The listing builds one solid part. Answer for the finished solid, in the listing's coordinates (mm). A direction names the side the tool comes from. Round coordinates to 2 decimals unless told otherwise and drop trailing zeros. Loops run counter-clockwise (first coordinate to the right, second up) from the corner with the lowest first, then second, coordinate; pieces in that order, holes last. Notation, with made-up numbers: (32, 59) - (42, 59) arc R13 cw to (42, 65) - close; hole circle Ø5 at (-15.75, -5). An arc over 180 degrees is marked (long way). Write item = value, one per line. Start each with the question number.
1) Section A-A, the plane x = -52 is taken. Determine the outline of the cut face in (y, z).
2) Section C-C, the plane z = 27 is taken. Determine the outline of the cut face in (x, y).
3) Given pin 1 Ø1.6 at (y, z) = (1, -34) entering from -X; pin 2 Ø1 at (x, z) = (-32, 20) entering from +Y; pin 3 Ø1.2 at (x, y) = (18.5, 1) entering from +Z; pin 4 Ø2 at (x, z) = (41, -18) entering from -Y, each flat-ended and moving along its own axis, determine where each tip first touches the part or whether it passes through.
4) A tool of negligible diameter and unlimited length cuts with its end or side. For faces 1 (the flat face through (42, 3.5, 36)), 2 (the flat face through (44.2, 1.7, -33)), 3 (the flat face through (52, 30, -35)), 4 (the flat face through (-50, 3.5, -36)), from which of +Z, -Z, +X, -X, +Y, -Y can it reach the whole face along a straight path? Write none if from no direction.
5) Section B-B, the plane y = 6 is taken. Determine the outline of the cut face in (x, z), and give its area (3 significant figures).
6) Section D-D, the plane y = 13.5 is taken. Give the number of separate pieces and of enclosed holes in the cut face, and give its area (3 significant figures).
7) Straight lines are drawn through the part: line 1 along Y through (x, z) = (-52, -36); line 2 along X through (y, z) = (38, 4.5); line 3 along X through (y, z) = (13, -36). For each, find the intervals that lie inside material, in ascending order.
8) For a pull along Y with two mould halves and no side action, classify faces 5 (the flat face through (46, 30, 0)), 6 (the flat face through (-42, 3.5, 36)), 7 (the cylindrical face through (-49.69, 12.54, -35.74)), 8 (the flat face through (-45, 57.5, -6)) as released by +Y, released by -Y, zero draft, split by the parting line, or undercut.
from build123d import *

# Parameters (mm, degrees)
SKETCH1_W                    = 89
SKETCH1_H                    = 70
BASE_FLANGE1_DEPTH           = 1.5
EDGE_FLANGE1_STRIP_W         = 10
EDGE_FLANGE1_STRIP_H         = 1.5
EDGE_FLANGE1_STRIP_CUT_DEPTH = 70
EDGE_FLANGE1_DEPTH           = 70
EDGE_FLANGE2_DEPTH           = 57.5
EDGE_FLANGE2_2_DEPTH         = 3.5
EDGE_FLANGE2_START           = 3.5
EDGE_FLANGE2_3_DEPTH         = 54
EDGE_FLANGE3_DEPTH           = 57.5
EDGE_FLANGE3_2_DEPTH         = 3.5
EDGE_FLANGE3_START           = 3.5
EDGE_FLANGE3_3_DEPTH         = 54
SKETCH16_R                   = 2.5
CUT_EXTRUDE1_DEPTH           = 10


# Read off the part's stored shape, not the designer's step: Edge-Flange2, Edge-Flange3
# Sheet-metal steps are written as plain solids
with BuildPart() as part:
    # Sketch1 → Base-Flange1 (new body)
    with BuildSketch(Plane(origin=(0, 0, 0), x_dir=(1, 0, 0), z_dir=(0, 1, 0))):
        Rectangle(SKETCH1_W, SKETCH1_H)
    extrude(amount=BASE_FLANGE1_DEPTH)

    # Edge-Flange1 strip (across the edge) → Edge-Flange1 strip cut (cut)
    with BuildSketch(Plane(origin=(-44.5, 1.5, -35), x_dir=(1, 0, 0), z_dir=(0, 0, 1))):
        with Locations((-3, -0.75)):
            Rectangle(EDGE_FLANGE1_STRIP_W, EDGE_FLANGE1_STRIP_H)
    edge_flange1_strip_cut = extrude(amount=EDGE_FLANGE1_STRIP_CUT_DEPTH, mode=Mode.SUBTRACT)

    # Edge-Flange1 section (across the edge) → Edge-Flange1 (add)
    with BuildSketch(Plane(origin=(-44.5, 1.5, -35), x_dir=(1, 0, 0), z_dir=(0, 0, 1))):
        with BuildLine():
            Line((-1.5, 2), (-1.5, 56))
            Line((-1.5, 56), (0, 56))
            Line((0, 56), (0, 2))
            ThreePointArc((0, 2), (0.585786438, 0.585786438), (2, 0))
            Line((2, 0), (2, -1.5))
            ThreePointArc((2, -1.5), (-0.474873734, -0.474873734), (-1.5, 2))
        make_face()
    edge_flange1 = extrude(amount=EDGE_FLANGE1_DEPTH)

    # Mirror1: Edge-Flange1 strip cut, Edge-Flange1 across plane
    add(edge_flange1_strip_cut.mirror(Plane(origin=(0, 0, 0), x_dir=(0, 0, 1), z_dir=(1, 0, 0))), mode=Mode.SUBTRACT)
    add(edge_flange1.mirror(Plane(origin=(0, 0, 0), x_dir=(0, 0, 1), z_dir=(1, 0, 0))))

    # Edge-Flange2 outline → Edge-Flange2 (cut)
    with BuildSketch(Plane(origin=(0, 0, 0), x_dir=(1, 0, 0), z_dir=(0, 1, 0))):
        with BuildLine():
            Line((45.127718677, 35), (42.5, 35))
            Line((42.5, 35), (42.5, 33))
            Line((42.5, 33), (44.5, 33))
            ThreePointArc((44.5, 33), (44.66061498, 34.048097173), (45.127718677, 35))
        make_face()
    edge_flange2 = extrude(amount=EDGE_FLANGE2_DEPTH, mode=Mode.SUBTRACT)

    # Edge-Flange2 2 outline → Edge-Flange2 2 (cut)
    with BuildSketch(Plane(origin=(0, 0, 0), x_dir=(1, 0, 0), z_dir=(0, 1, 0))):
        with BuildLine():
            ThreePointArc((45.127718677, 35), (44.66061498, 34.048097173), (44.5, 33))
            Line((44.5, 33), (46, 33))
            ThreePointArc((46, 33), (46.585786438, 34.414213562), (48, 35))
            Line((48, 35), (56, 35))
            Line((56, 35), (56, 36.5))
            Line((56, 36.5), (48, 36.5))
            ThreePointArc((48, 36.5), (46.379814826, 36.102418411), (45.127718677, 35))
        make_face()
    edge_flange2_2 = extrude(amount=EDGE_FLANGE2_2_DEPTH, mode=Mode.SUBTRACT)

    # Edge-Flange2 3 outline → Edge-Flange2 3 (add)
    with BuildSketch(Plane(origin=(0, 0, 0), x_dir=(1, 0, 0), z_dir=(0, 1, 0)).offset(EDGE_FLANGE2_START)):
        with BuildLine():
            ThreePointArc((45.127718677, 35), (44.66061498, 34.048097173), (44.5, 33))
            Line((44.5, 33), (46, 33))
            ThreePointArc((46, 33), (46.585786438, 34.414213562), (48, 35))
            Line((48, 35), (56, 35))
            Line((56, 35), (56, 36.5))
            Line((56, 36.5), (48, 36.5))
            ThreePointArc((48, 36.5), (46.379814826, 36.102418411), (45.127718677, 35))
        make_face()
    edge_flange2_3 = extrude(amount=EDGE_FLANGE2_3_DEPTH)

    # Mirror2: Edge-Flange2, Edge-Flange2 2, Edge-Flange2 3 across plane
    add(edge_flange2.mirror(Plane(origin=(0, 0, 0), x_dir=(0, 0, 1), z_dir=(1, 0, 0))), mode=Mode.SUBTRACT)
    add(edge_flange2_2.mirror(Plane(origin=(0, 0, 0), x_dir=(0, 0, 1), z_dir=(1, 0, 0))), mode=Mode.SUBTRACT)
    add(edge_flange2_3.mirror(Plane(origin=(0, 0, 0), x_dir=(0, 0, 1), z_dir=(1, 0, 0))))

    # Edge-Flange3 outline → Edge-Flange3 (cut)
    with BuildSketch(Plane(origin=(0, 0, 0), x_dir=(1, 0, 0), z_dir=(0, 1, 0))):
        with BuildLine():
            ThreePointArc((-44.5, -33), (-43.914213562, -34.414213562), (-42.5, -35))
            Line((-42.5, -35), (-42.5, -33))
            Line((-42.5, -33), (-44.5, -33))
        make_face()
        with BuildLine():
            ThreePointArc((-45.372281323, -35), (-45.83938502, -34.048097173), (-46, -33))
            Line((-46, -33), (-46, -35))
            Line((-46, -35), (-45.372281323, -35))
        make_face()
    edge_flange3 = extrude(amount=EDGE_FLANGE3_DEPTH, mode=Mode.SUBTRACT)

    # Edge-Flange3 2 outline → Edge-Flange3 2 (cut)
    with BuildSketch(Plane(origin=(0, 0, 0), x_dir=(1, 0, 0), z_dir=(0, 1, 0))):
        with BuildLine():
            ThreePointArc((-42.5, -35), (-43.914213562, -34.414213562), (-44.5, -33))
            Line((-44.5, -33), (-46, -33))
            ThreePointArc((-46, -33), (-45.83938502, -34.048097173), (-45.372281323, -35))
            Line((-45.372281323, -35), (-42.5, -35))
        make_face()
    edge_flange3_2 = extrude(amount=EDGE_FLANGE3_2_DEPTH, mode=Mode.SUBTRACT)

    # Edge-Flange3 3 outline → Edge-Flange3 3 (add)
    with BuildSketch(Plane(origin=(0, 0, 0), x_dir=(1, 0, 0), z_dir=(0, 1, 0)).offset(EDGE_FLANGE3_START)):
        with BuildLine():
            Line((-44.5, -33), (-44.5, -35))
            Line((-44.5, -35), (-45.372281323, -35))
            ThreePointArc((-45.372281323, -35), (-44.120185174, -36.102418411), (-42.5, -36.5))
            Line((-42.5, -36.5), (-38.5, -36.5))
            Line((-38.5, -36.5), (-38.5, -35))
            Line((-38.5, -35), (-42.5, -35))
            ThreePointArc((-42.5, -35), (-43.914213562, -34.414213562), (-44.5, -33))
        make_face()
    edge_flange3_3 = extrude(amount=EDGE_FLANGE3_3_DEPTH)

    # Mirror3: Edge-Flange3, Edge-Flange3 2, Edge-Flange3 3 across plane
    add(edge_flange3.mirror(Plane(origin=(0, 0, 0), x_dir=(0, 0, 1), z_dir=(1, 0, 0))), mode=Mode.SUBTRACT)
    add(edge_flange3_2.mirror(Plane(origin=(0, 0, 0), x_dir=(0, 0, 1), z_dir=(1, 0, 0))), mode=Mode.SUBTRACT)
    add(edge_flange3_3.mirror(Plane(origin=(0, 0, 0), x_dir=(0, 0, 1), z_dir=(1, 0, 0))))

    # Sketch16 → Cut-Extrude1 (cut)
    with BuildSketch(Plane.XY.offset(-35)):
        with Locations((52, 47.5)):
            Circle(SKETCH16_R)
        with Locations((52, 13.5)):
            Circle(SKETCH16_R)
        with Locations((-52, 47.5)):
            Circle(SKETCH16_R)
        with Locations((-52, 13.5)):
            Circle(SKETCH16_R)
    extrude(amount=-CUT_EXTRUDE1_DEPTH, mode=Mode.SUBTRACT)


solid = part.part
Geometry check:
q1.outline = (3.5, -36.5) - (11, -36.5) - (11, -35) - (3.5, -35) - close; (16, -36.5) - (45, -36.5) - (45, -35) - (16, -35) - close; (50, -36.5) - (57.5, -36.5) - (57.5, -35) - (50, -35) - close
q2.outline = (-46, 3.5) arc R3.5 ccw to (-42.5, 0) - (42.5, 0) arc R3.5 ccw to (46, 3.5) - (46, 57.5) - (44.5, 57.5) - (44.5, 3.5) arc R2 cw to (42.5, 1.5) - (-42.5, 1.5) arc R2 cw to (-44.5, 3.5) - (-44.5, 57.5) - (-46, 57.5) - close
q3.pin_1 = -42.5
q3.pin_2 = 1.5
q3.pin_3 = 35
q3.pin_4 = 0
q4.face_1 = +Z, +X, -X, -Y
q4.face_2 = -Z, +X, -Y
q4.face_3 = +Z, +X, +Y, -Y
q4.face_4 = -Z, +X, -X, -Y
q5.outline = (-56, -36.5) - (-48, -36.5) arc R3.5 ccw to (-44.5, -33) - (-44.5, 33) arc R2 cw to (-42.5, 35) - (-38.5, 35) - (-38.5, 36.5) - (-42.5, 36.5) arc R3.5 ccw to (-46, 33) - (-46, -33) arc R2 cw to (-48, -35) - (-56, -35) - close; (38.5, 35) - (42.5, 35) arc R2 cw to (44.5, 33) - (44.5, -33) arc R3.5 ccw to (48, -36.5) - (56, -36.5) - (56, -35) - (48, -35) arc R2 cw to (46, -33) - (46, 33) arc R3.5 ccw to (42.5, 36.5) - (38.5, 36.5) - close
q5.area = 260 mm2
q6.separate_pieces = 4
q6.enclosed_holes = 0
q6.area = 245 mm2
q7.line_1 = 3.5 to 11, 16 to 45, 50 to 57.5
q7.line_2 = -46 to -44.5, 44.5 to 46
q7.line_3 = -56 to -54.45, -49.55 to -46.2, 46.2 to 49.55, 54.45 to 56
q8.face_5 = zero draft
q8.face_6 = released by -Y
q8.face_7 = undercut
q8.face_8 = released by +Y
